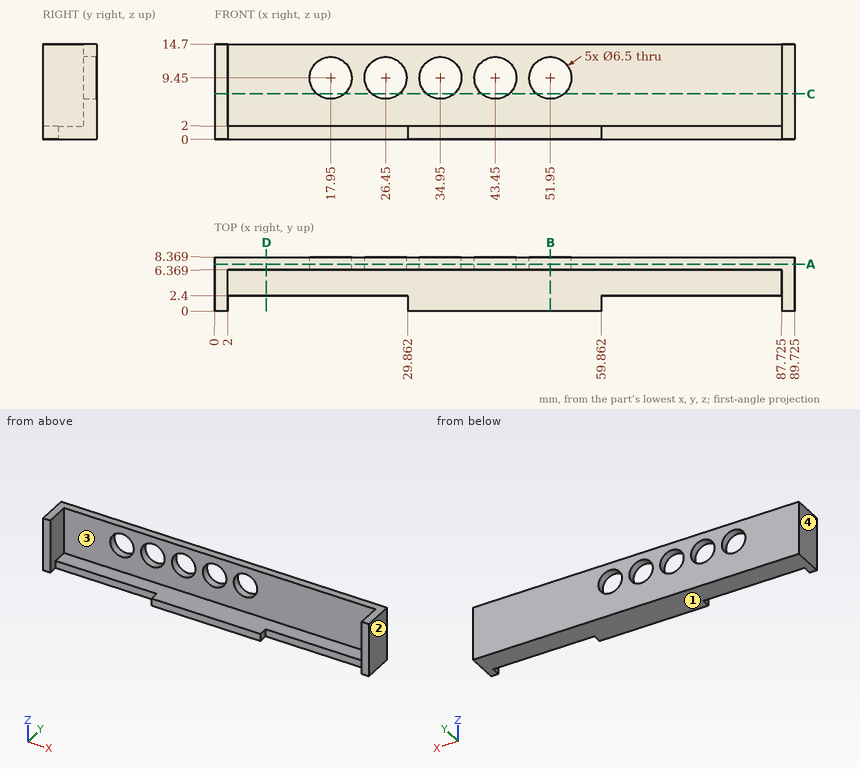
Input: dimensioned drawing with shaded views. Units: mm. Origin: part minimum x, y, z. Coordinates: 2 decimals unless noted, no trailing zeros. Order: outer loops, then holes, each group sorted by start corner. A loop starts at its lowest first (then second) coordinate and runs counter-clockwise, first axis right, second up. Notation, with made-up numbers: (1.25, 48.25) - (25.25, 48.25) arc R22 ccw to (25.25, 72.25) - close; hole circle Ø6 at (32, -18.75). An arc over 180 degrees is marked (long way). Return JSON: item names as keys, results as strings. Group by question number.
1. Cut plane A-A (y = 7.25). Count the separate pieces of the cut face and the enclosed holes in it, plus the area to 3 significant figures.
2. Material intervals for line 1 along X through (y, z) = (8.05, 9.45) (1 decimal); line 2 along X through (y, z) = (6, 12.25) (1 decimal); line 3 along Y through (x, z) = (64, 5.75), sorted ascending. Write a range as [from, to].
3. Cut plane C-C (z = 7). Output: boundary loops of the cut face in (x, y) (1 decimal), plus the area to 3 significant figures.
4. Pull-direction query (X, two-part tool) for the marked faces 1, 2, 3 and 4; classes: pulls with the +X half, pulls with the -X half, needs draft (parallel to the pull), parting line crosses it, or undercut.
5. Pin query (flat end, axial travel): pin 1 (1.5 mm diameter, centred on x = 42.5, z = 4.5, fed in from -Y); pin 2 (2 mm diameter, centred on x = 71.5, z = 0.5, fed in from -Y); pin 3 (5 mm diameter, centred on x = 26.45, z = 9.45, fed in from -Y); pin 4 (1 mm diameter, centred on x = 41.5, y = 1, fed in from +Z). Return the tip coordinate at first contact, or that it passes through.
6. Cut plane D-D (x = 8). Output: boundary loops of the cut face in (y, z).
7. Cut plane B-B (x = 51.95). Output: boundary loops of the cut face in (y, z).
Resolved:
{
 "1": {"separate pieces": "1", "enclosed holes": "5", "area": "1,150 mm²"},
 "2": {"line 1": "x = [0, 14.7], [21.2, 23.2], [29.7, 31.7], [38.2, 40.2], [46.7, 48.7], [55.2, 89.7]", "line 2": "x = [0, 2], [87.7, 89.7]", "line 3": "y = [6.37, 8.37]"},
 "3": {"outline": "(0, 0) - (2, 0) - (2, 6.4) - (15.8, 6.4) - (15.8, 8.4) - (0, 8.4) - close; (20.1, 6.4) - (24.3, 6.4) - (24.3, 8.4) - (20.1, 8.4) - close; (28.6, 6.4) - (32.8, 6.4) - (32.8, 8.4) - (28.6, 8.4) - close; (37.1, 6.4) - (41.3, 6.4) - (41.3, 8.4) - (37.1, 8.4) - close; (45.6, 6.4) - (49.8, 6.4) - (49.8, 8.4) - (45.6, 8.4) - close; (54.1, 6.4) - (87.7, 6.4) - (87.7, 0) - (89.7, 0) - (89.7, 8.4) - (54.1, 8.4) - close", "area": "162 mm²"},
 "4": {"face 1": "needs draft", "face 2": "pulls with the +X half", "face 3": "undercut", "face 4": "pulls with the -X half"},
 "5": {"pin 1": "stops at y = 6.37", "pin 2": "stops at y = 2.4", "pin 3": "passes through", "pin 4": "stops at z = 2"},
 "6": {"outline": "(2.4, 0) - (8.37, 0) - (8.37, 14.7) - (6.37, 14.7) - (6.37, 2) - (2.4, 2) - close"},
 "7": {"outline": "(0, 0) - (8.37, 0) - (8.37, 6.2) - (6.37, 6.2) - (6.37, 2) - (0, 2) - close; (6.37, 12.7) - (8.37, 12.7) - (8.37, 14.7) - (6.37, 14.7) - close"}
}
